Autodesk Inventor part; units mm, degrees
ref_plane "Piano iniziale" through (0, 0, 0) normal (0, 0, 1) x (1, 0, 0)
ref_plane "Piano finale" through (0, 0, 700) normal (0, 0, 1) x (1, 0, 0)
ref_plane "YZ Plane" through (0, 0, 0) normal (1, 0, 0) x (0, 1, 0)
ref_plane "Piano iniziale" through (0, 0, 0) normal (0, 0, 1) x (1, 0, 0)
ref_plane "Piano finale" through (0, 0, 700) normal (0, 0, 1) x (1, 0, 0)
sketch "Schizzo" plane through (0, 0, 0) normal (0, 0, 1) x (1, 0, 0)
  line L0 (-20, -16) -> (-20, 16)
  line L1 (-16, 20) -> (16, 20)
  line L2 (20, 16) -> (20, -16)
  line L3 (16, -20) -> (-16, -20)
  arc A0 (-20, -16) -> (-16, -20) centre (-16, -16) ccw
  arc A1 (20, 16) -> (16, 20) centre (16, 16) ccw
  arc A2 (-16, 20) -> (-20, 16) centre (-16, 16) ccw
  arc A3 (16, -20) -> (20, -16) centre (16, -16) ccw
  arc A4 (-16, 18) -> (-18, 16) centre (-16, 16) ccw
  line L4 (-16, 18) -> (16, 18)
  arc A5 (18, 16) -> (16, 18) centre (16, 16) ccw
  line L5 (18, 16) -> (18, -16)
  arc A6 (16, -18) -> (18, -16) centre (16, -16) ccw
  line L6 (16, -18) -> (-16, -18)
  arc A7 (-18, -16) -> (-16, -18) centre (-16, -16) ccw
  line L7 (-18, -16) -> (-18, 16)
  line L8 (0, 29.1598) -> (0, -29.1598) construction
  line L9 (-29.1598, 0) -> (29.1598, 0) construction
  dimension "d7" = 4
  dimension "d9" = 40
  dimension "d11" = 40
  dimension "d12" = 2
  dimension "d15" = 20
  dimension "d16" = 20
extrude "Corpo" add sketch "Schizzo" along normal up to surface (700 mm away) from surface at 0
sketch "Sketch3" plane through (0, 0, 0) normal (0, 0, 1) x (1, 0, 0)
  line L0 (0, 0) -> (10, 0)
ref_plane "Work Plane3" through (0, 0, 0) normal (0, -1, 0) x (1, 0, 0)
sketch "Sketch4" plane through (0, 0, 0) normal (0, -1, 0) x (1, 0, 0)
  line L0 (-2, 0) -> (12, 0)
  line L1 (-2, 700) -> (12, 700)
  dimension "d18" = 700
sketch "Schizzo5" plane through (-16, -20, 0) normal (0, -1, 0) x (1, 0, 0)
  line L0 (-4, 0) -> (-4, 700)
  line L1 (-4, 0) -> (0, 0)
  line L2 (-4, 700) -> (0, 700)
  line L3 (-4, 700) -> (0, 700)
  line L4 (-4, 700) -> (46.6766, 649.3234)
  line L5 (-4, 700) -> (67.6675, 700) construction
  line L6 (46.6766, 649.3234) -> (46.6766, 733.8871)
  line L7 (46.6766, 733.8871) -> (-4, 700)
  line L8 (-4, 0) -> (55.8193, 59.8193)
  line L9 (-4, 0) -> (80.5973, 0) construction
  line L10 (55.8193, 59.8193) -> (55.8193, -51.0015)
  line L11 (55.8193, -51.0015) -> (-4, 0)
  point P0 (16, 0)
  dimension "d19" = 45
  dimension "d20" = 45
extrude "Estrusione2" cut sketch "Schizzo5" against normal up to next
sketch "Schizzo6" plane through (20, -16, 660) normal (1, 0, 0) x (0, 0, -1)
  circle A0 centre (230, 8.5) radius 5
  circle A1 centre (545, 8.5) radius 5
  circle A2 centre (335, 8.5) radius 5
  circle A3 centre (440, 8.5) radius 5
  line L0 (0, 0) -> (0, 32)
  line L1 (620, 32) -> (0, 32)
  line L2 (620, 0) -> (620, 32)
  line L3 (620, 0) -> (0, 0)
  point P0 (660, 16)
hole "Foro1" at (20, -7.5, 115) at (20, -7.5, 220) at (20, -7.5, 325) at (20, -7.5, 430) direction (-1, 0, 0) diameter 10 depth 8 tip angle 118
equation "\"d7\" = G_IR"
equation "\"d9\" = G_W"
equation "\"d11\" = G_H"
equation "\"d12\" = G_T"
equation "\"d15\" = 0.5 * d9"
equation "\"d16\" = 0.5 * d11"
equation "\"d3\" = G_L"
equation "\"G_W\" = 40"
equation "\"G_H\" = 40"
equation "\"G_T\" = 2"
equation "\"G_IR\" = 4"
equation "\"G_L\" = d18"
equation "\"G_OFFSET_START\" = 0"
equation "\"G_OFFSET_END\" = 0"
properties part number "ISO 10799-2 - 40x40x2 - 700" material "Acciaio, Dolce"
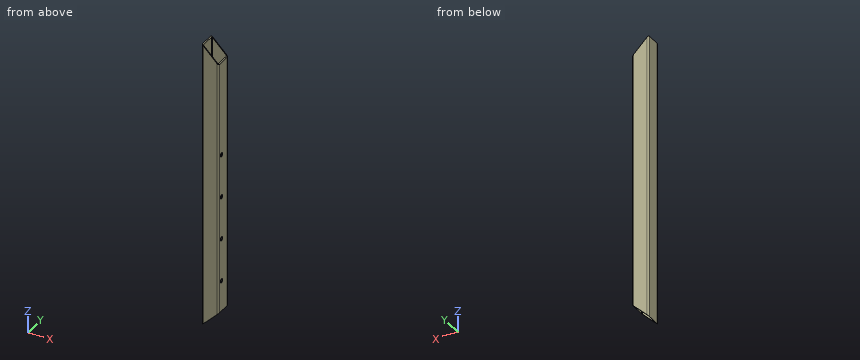
Model file for the job. Use its own axes, mm. Give positions to 0.01 mm unless a question says otherwise; leave off trailing zeros. Loops run counter-clockwise (first coordinate to the right, second up) from the corner with the lowest first, then second, coordinate; pieces in that order, holes last. Notation, with made-up numbers: (15.25, -14) -> (56.25, -14) arc R18 cw to (56.25, -9) -> close; hole circle Ø7 at (58.25, 3.5). An arc over 180 degrees is marked (long way). Use a Markdown table: item, result. Add a question column.
(1) Slice it at A-A on y = 10. List the corners of the cut face in (x, z), and give its area (3 significant figures).
(2) Slice it at C-C on z = 575. List the corners of the cut face in (x, y).
(3) Wall check: line 1 along X through (y, z) = (10, 410); line 2 along Z through (x, y) = (19.35, -7.5). Give the ranges that are in metal, low to high.
(4) Drop flat-ended pins along their axis: pin 1 Ø6 at (y, z) = (-7.5, 115) entering from +X; pin 2 Ø8 at (x, y) = (8.5, -14.5) entering from +Z; pin 3 Ø10 at (x, y) = (-6, 14) entering from +Z; pin 4 Ø10 at (x, y) = (-8.5, 1.5) entering from -Z. Give the stop position or say it passes through.
(5) Slice it at B-B on x = 1.5. List the corners of the cut face in (y, z), and give its area (3 significant figures).
Filled sheet:
| question | item | result |
|---|---|---|
| 1 | outline | (-20, 0) -> (-18, 2) -> (-18, 698) -> (-20, 700) -> close; (18, 38) -> (20, 40) -> (20, 660) -> (18, 662) -> close |
| 1 | area | 2,640 mm2 |
| 2 | outline | (-20, -16) arc R4 ccw to (-16, -20) -> (16, -20) arc R4 ccw to (20, -16) -> (20, 16) arc R4 ccw to (16, 20) -> (-16, 20) arc R4 ccw to (-20, 16) -> close; hole (-18, -16) arc R2 ccw to (-16, -18) -> (16, -18) arc R2 ccw to (18, -16) -> (18, 16) arc R2 ccw to (16, 18) -> (-16, 18) arc R2 ccw to (-18, 16) -> close |
| 3 | line 1 | -20 to -18, 18 to 20 |
| 3 | line 2 | 39.35 to 110, 120 to 215, 225 to 320, 330 to 425, 435 to 660.65 |
| 4 | pin 1 | x = -18 |
| 4 | pin 2 | z = 673.44 |
| 4 | pin 3 | z = 689 |
| 4 | pin 4 | through |
| 5 | outline | (-20, 21.5) -> (-18, 21.5) -> (-18, 678.5) -> (-20, 678.5) -> close; (18, 21.5) -> (20, 21.5) -> (20, 678.5) -> (18, 678.5) -> close |
| 5 | area | 2,630 mm2 |
